```python
from build123d import *

# Parameters (mm, degrees)
BOSS_EXTRUDE1_DEPTH     = 38.1
SKETCH3_R               = 3.175
BOSS_EXTRUDE3_DEPTH     = 19.05
CUT_EXTRUDE1_DEPTH      = 39.418677326
CUT_EXTRUDE1_DEPTH_BACK = 39.418677326
SKETCH4_R               = 0.79375
CUT_EXTRUDE4_DEPTH      = 8.636
SKETCH6_OUTSIDE_W       = 20.904
SKETCH6_OUTSIDE_H       = 20.248
SKETCH6_OUTSIDE_R       = 2.667
CUT_EXTRUDE5_DEPTH      = 0.762
SKETCH9_OUTSIDE_W       = 20.904
SKETCH9_OUTSIDE_H       = 20.248
SKETCH9_OUTSIDE_R       = 2.667
CUT_EXTRUDE6_DEPTH      = 0.762
SKETCH10_OUTSIDE_W      = 20.904
SKETCH10_OUTSIDE_H      = 20.248
SKETCH10_OUTSIDE_R      = 2.667
CUT_EXTRUDE7_DEPTH      = 0.762


with BuildPart() as part:
    # Sketch1 → Boss-Extrude1 (new body)
    with BuildSketch(Plane(origin=(0, 0, 0), x_dir=(0, 0, -1), z_dir=(1, 0, 0))):
        Polygon((2.105028301, -3.00161443), (3.651988499, 0.32220077), (1.546960198, 3.323815199), (-2.105028301, 3.00161443), (-3.651988499, -0.32220077), (-1.546960198, -3.323815199), align=None)
    extrude(amount=BOSS_EXTRUDE1_DEPTH)

    # Sketch3 → Boss-Extrude3 (add)
    with BuildSketch(Plane.ZY):
        with Locations(Location((0, 0, 0), (0, 0, 204.958070598))):
            Circle(SKETCH3_R)
    extrude(amount=BOSS_EXTRUDE3_DEPTH)

    # Sketch4 → Cut-Extrude1 (cut, two sides: drawn at the far end of the back side and taken through both)
    with BuildSketch(Plane(origin=(0, 0, 0), x_dir=(1, 0, 0), z_dir=(0, 1, 0)).offset(-CUT_EXTRUDE1_DEPTH_BACK)):
        with Locations(Location((-16.51, 0, 0), (0, 0, 90))):
            Circle(SKETCH4_R)
    extrude(amount=CUT_EXTRUDE1_DEPTH + CUT_EXTRUDE1_DEPTH_BACK, mode=Mode.SUBTRACT)

    # Sketch5 → Cut-Extrude4 (cut)
    with BuildSketch(Plane(origin=(38.1, 0, 0), x_dir=(0, 0, -1), z_dir=(1, 0, 0))):
        with BuildLine():
            Line((-2.878508392, 1.339706848), (-2.105028301, 3.00161443))
            ThreePointArc((-2.105028301, 3.00161443), (-3.323815199, 1.546960198), (-3.651988499, -0.32220077))
            Line((-3.651988499, -0.32220077), (-2.878508392, 1.339706848))
        make_face()
        with BuildLine():
            Line((-2.878508392, 1.339706848), (-3.651988499, -0.32220077))
            Line((-3.651988499, -0.32220077), (-2.599474334, -1.823008005))
            ThreePointArc((-2.599474334, -1.823008005), (-3.162714814, -0.279034054), (-2.878508392, 1.339706848))
        make_face()
        with BuildLine():
            ThreePointArc((-3.651988499, -0.32220077), (-3.00161443, -2.105028301), (-1.546960198, -3.323815199))
            Line((-1.546960198, -3.323815199), (-2.599474334, -1.823008005))
            Line((-2.599474334, -1.823008005), (-3.651988499, -0.32220077))
        make_face()
        with BuildLine():
            Line((-2.599474334, -1.823008005), (-1.546960198, -3.323815199))
            Line((-1.546960198, -3.323815199), (0.279034067, -3.162714813))
            ThreePointArc((0.279034067, -3.162714813), (-1.339706811, -2.878508409), (-2.599474334, -1.823008005))
        make_face()
        with BuildLine():
            ThreePointArc((-1.546960198, -3.323815199), (0.32220077, -3.651988499), (2.105028301, -3.00161443))
            Line((2.105028301, -3.00161443), (0.279034067, -3.162714813))
            Line((0.279034067, -3.162714813), (-1.546960198, -3.323815199))
        make_face()
        with BuildLine():
            Line((0.279034067, -3.162714813), (2.105028301, -3.00161443))
            Line((2.105028301, -3.00161443), (2.878508392, -1.339706848))
            ThreePointArc((2.878508392, -1.339706848), (1.823007983, -2.59947435), (0.279034067, -3.162714813))
        make_face()
        with BuildLine():
            ThreePointArc((2.105028301, -3.00161443), (3.252555442, -1.69166085), (3.666174209, 0))
            ThreePointArc((3.666174209, 0), (3.662626065, 0.16125645), (3.651988499, 0.32220077))
            Line((3.651988499, 0.32220077), (2.878508392, -1.339706848))
            Line((2.878508392, -1.339706848), (2.105028301, -3.00161443))
        make_face()
        with BuildLine():
            Line((2.878508392, -1.339706848), (3.651988499, 0.32220077))
            Line((3.651988499, 0.32220077), (2.599474407, 1.823007901))
            ThreePointArc((2.599474407, 1.823007901), (3.027701789, 0.955848774), (3.175, 0))
            ThreePointArc((3.175, 0), (3.09999106, -0.686061534), (2.878508392, -1.339706848))
        make_face()
        with BuildLine():
            Line((2.599474407, 1.823007901), (3.651988499, 0.32220077))
            ThreePointArc((3.651988499, 0.32220077), (3.00161443, 2.105028301), (1.546960198, 3.323815199))
            Line((1.546960198, 3.323815199), (2.599474407, 1.823007901))
        make_face()
        with BuildLine():
            Line((2.599474407, 1.823007901), (1.546960198, 3.323815199))
            Line((1.546960198, 3.323815199), (-0.279034067, 3.162714813))
            ThreePointArc((-0.279034067, 3.162714813), (1.339706869, 2.878508382), (2.599474407, 1.823007901))
        make_face()
        with BuildLine():
            Line((-0.279034067, 3.162714813), (1.546960198, 3.323815199))
            ThreePointArc((1.546960198, 3.323815199), (-0.32220077, 3.651988499), (-2.105028301, 3.00161443))
            Line((-2.105028301, 3.00161443), (-0.279034067, 3.162714813))
        make_face()
        with BuildLine():
            Line((-0.279034067, 3.162714813), (-2.105028301, 3.00161443))
            Line((-2.105028301, 3.00161443), (-2.878508392, 1.339706848))
            ThreePointArc((-2.878508392, 1.339706848), (-1.823007983, 2.59947435), (-0.279034067, 3.162714813))
        make_face()
    extrude(amount=-CUT_EXTRUDE4_DEPTH, mode=Mode.SUBTRACT)

    # Sketch6 outside → Cut-Extrude5 (cut)
    with BuildSketch(Plane(origin=(37.084, 0, 0), x_dir=(0, 0, -1), z_dir=(1, 0, 0))):
        Rectangle(SKETCH6_OUTSIDE_W, SKETCH6_OUTSIDE_H)
        with Locations(Location((0, 0, 0), (0, 0, 180))):
            Circle(SKETCH6_OUTSIDE_R, mode=Mode.SUBTRACT)
    extrude(amount=CUT_EXTRUDE5_DEPTH, mode=Mode.SUBTRACT)

    # Sketch9 outside → Cut-Extrude6 (cut)
    with BuildSketch(Plane.ZY.offset(8.128)):
        Rectangle(SKETCH9_OUTSIDE_W, SKETCH9_OUTSIDE_H)
        Circle(SKETCH9_OUTSIDE_R, mode=Mode.SUBTRACT)
    extrude(amount=CUT_EXTRUDE6_DEPTH, mode=Mode.SUBTRACT)

    # Sketch10 outside → Cut-Extrude7 (cut)
    with BuildSketch(Plane.ZY.offset(-13.97)):
        Rectangle(SKETCH10_OUTSIDE_W, SKETCH10_OUTSIDE_H)
        with Locations(Location((0, 0, 0), (0, 0, 180))):
            Circle(SKETCH10_OUTSIDE_R, mode=Mode.SUBTRACT)
    extrude(amount=CUT_EXTRUDE7_DEPTH, mode=Mode.SUBTRACT)


solid = part.part
```
The model under review builds one solid part; all positions refer to its coordinate system, in mm. A direction names the side the tool comes from. Round coordinates to 2 decimals unless told otherwise and drop trailing zeros. Order: outer loops, then holes, each group sorted by start corner. A loop starts at its lowest first (then second) coordinate and runs counter-clockwise, first axis right, second up.
(1) Take a section at B-B, the plane x = -16.51. State the section outline as (y, z) points (3 decimals), plus the area to 3 significant figures.
Working result:
outline: (-3.074, -0.794) arc R3.175 ccw to (3.074, -0.794) - close; (-3.074, 0.794) - (3.074, 0.794) arc R3.175 ccw to start
area: 21.7 mm2
(2) For P1, Ø1, axis at x = -4.5, y = -1, coming from the -Z side; P2, Ø2.5, axis at x = -16.51, z = 0, coming from the +Y side (3 decimals); P3, Ø2, axis at x = -6.5, z = 3, coming from the -Y side, all flat-tipped, find the tip position at first contact; note any pin that passes through.
Working result:
P1: stops at z = -3.14
P2: stops at y = 3.175
P3: stops at y = -2.47
(3) Tool access review of faces 1 (the face through (13.97, -3, 0)), 2 (the face through (29.464, 2.7, 2)), 3 (the face through (-4.007, -2.142, -2.343)): name each direction out of +Z, -Z, +X, -X, +Y, -Y from which nothing blocks a thin tool from reaching the whole face with its end or side.
Working result:
face 1: none
face 2: +Z, +X, +Y
face 3: -X
(4) Take a section at C-C, the plane x = 6.5. State the section outline as (y, z) points.
Working result:
outline: (-3.32, 1.55) - (-3, -2.11) - (0.32, -3.65) - (3.32, -1.55) - (3, 2.11) - (-0.32, 3.65) - close
(5) Mouldability with a two-part tool opening along Z and no side actions: class faces 4 (the face through (29.464, -3.1, 1.4)), 5 (the face through (-15.735, -0.044, 0.172)), 6 (the face through (6.51, 1.36, 2.87)) as released by +Z, released by -Z, zero draft, split by the parting line, or undercut.
Working result:
face 4: zero draft
face 5: undercut
face 6: released by +Z
(6) Wall thickness on L1, parallel to X at y = 2.5, z = 2; L2, parallel to X at y = 0.5, z = 0; L3, parallel to Z at x = -16.51, y = 1.5: over which ranges is each line inside the solid? List them lowest first.
Working result:
L1: x = 0 to 13.21, 13.97 to 29.46
L2: x = -19.05 to -17.3, -15.72 to 38.1
L3: z = -2.8 to -0.79, 0.79 to 2.8
